Model file for the job. Use its own axes, mm. Face numbers are marked on the shaded views. A direction names the side the tool comes from. Round coordinates to 2 decimals unless told otherwise and drop trailing zeros. Loops run counter-clockwise (first coordinate to the right, second up) from the corner with the lowest first, then second, coordinate; pieces in that order, holes last. Notation, with made-up numbers: M 24,24.25 L 59,24.25 A20 cw 59,57.25 Z; hole C 4,-4.5 d5. An arc over 180 degrees is marked long. Answer in a Markdown table with one row per item.
from build123d import *

# Parameters (mm, degrees)
SKETCH_1_R          = 8
EXTRUDE_1_DEPTH     = 6
SKETCH_2_R          = 1.25
CUT_EXTRUDE_1_DEPTH = 3


with BuildPart() as part:
    # 草图1 → 凸台-拉伸1 (new body)
    with BuildSketch(Plane.XY):
        with BuildLine():
            Line((-3, -30), (-18, -30))
            Line((-18, -30), (-18, -27))
            Line((-18, -27), (-11.5, -27))
            Line((-11.5, -27), (-11.5, 0))
            ThreePointArc((-11.5, 0), (0, 11.5), (11.5, 0))
            Line((11.5, 0), (11.5, -27))
            Line((11.5, -27), (17.5, -27))
            Line((17.5, -27), (17.5, -30))
            Line((17.5, -30), (3, -30))
            Line((3, -30), (3, -33))
            Line((3, -33), (0, -33))
            Line((0, -33), (-3, -33))
            Line((-3, -33), (-3, -30))
        make_face()
        Circle(SKETCH_1_R, mode=Mode.SUBTRACT)
    extrude(amount=EXTRUDE_1_DEPTH)

    # 草图2 → 切除-拉伸1 (cut)
    with BuildSketch(Plane(origin=(0, -27, 0), x_dir=(1, 0, 0), z_dir=(0, 1, 0))):
        with Locations(Location((-14.5, -3, 0), (0, 0, 270))):
            Circle(SKETCH_2_R)
        with Locations(Location((14.5, -3, 0), (0, 0, 270))):
            Circle(SKETCH_2_R)
    extrude(amount=-CUT_EXTRUDE_1_DEPTH, mode=Mode.SUBTRACT)


solid = part.part
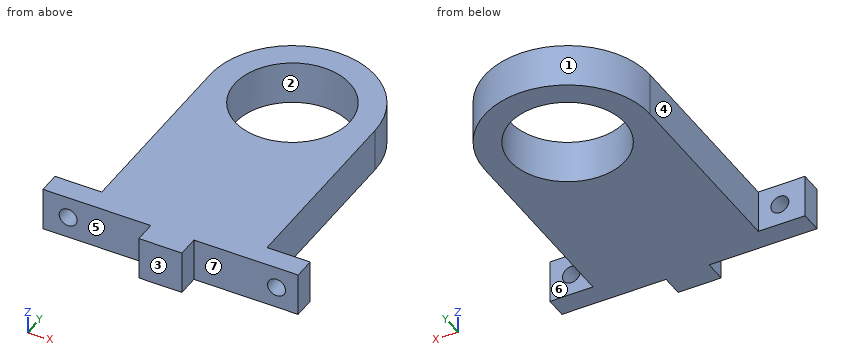
1. Wall check: probe 1 along X at (y, z) = (-29.3, 3); probe 2 along Y at (x, z) = (0, 3.25); probe 3 along X at (y, z) = (-25, 3.05). Give the ranges that are in metal, low to high.
Verdict:
| item | result |
|---|---|
| probe 1 | x = -18 to -15.75, -13.25 to 13.25, 15.75 to 17.5 |
| probe 2 | y = -33 to -8, 8 to 11.5 |
| probe 3 | x = -11.5 to 11.5 |
2. Mould opens along X. For the marked faces 1, 2 and 3 say: +X half, -X half, draft (parallel to the pull), parting line (faces both ways), or undercut.
Verdict:
| item | result |
|---|---|
| face 1 | parting line |
| face 2 | undercut |
| face 3 | draft |
3. Saw through at B-B (x = 0). Write the cut outline in (y, z).
Verdict:
| item | result |
|---|---|
| outline | M -33,0 L -8,0 L -8,6 L -33,6 Z; M 8,0 L 11.5,0 L 11.5,6 L 8,6 Z |
4. Saw through at A-A (z = 3). Write the cut outline in (x, y), and give its area (3 significant figures).
Verdict:
| item | result |
|---|---|
| outline | M -18,-30 L -15.75,-30 L -15.75,-27 L -18,-27 Z; M -13.25,-30 L -3,-30 L -3,-33 L 3,-33 L 3,-30 L 13.25,-30 L 13.25,-27 L 11.5,-27 L 11.5,0 A11.5 ccw -11.5,0 L -11.5,-27 L -13.25,-27 Z; M 15.75,-30 L 17.5,-30 L 17.5,-27 L 15.75,-27 Z; hole C 0,0 d16 |
| area | 737 mm² |
5. Saw through at D-D (y = -18.5). Write the cut outline in (x, z), and give its area (3 significant figures).
Verdict:
| item | result |
|---|---|
| outline | M -11.5,0 L 11.5,0 L 11.5,6 L -11.5,6 Z |
| area | 138 mm² |
6. Tool access for the marked faces 4, 5, 6 and 7: list every direction of +Z, -Z, +X, -X, +Y, -Y with a clear straight run to the whole face (end or side of a thin tool).
Verdict:
| item | result |
|---|---|
| face 4 | +Z, -Z, -X, +Y |
| face 5 | +Z, -Z, -X, -Y |
| face 6 | +Z, -Z, +X, +Y |
| face 7 | +Z, -Z, +X, -Y |
7. Saw through at C-C (y = -7). Write the cut outline in (x, z).
Verdict:
| item | result |
|---|---|
| outline | M -11.5,0 L -3.87,0 L -3.87,6 L -11.5,6 Z; M 3.87,0 L 11.5,0 L 11.5,6 L 3.87,6 Z |
8. Pin check, flat tips, straight feed: pin 1 (1.5 mm diameter, centred on y = -31.5, z = 3.5, fed in from +X); pin 2 (0.9 mm diameter, centred on y = -31, z = 4, fed in from -X); pin 3 (2 mm diameter, centred on y = -11.5, z = 5, fed in from -X). Stop position of each tip, or through.
Verdict:
| item | result |
|---|---|
| pin 1 | stops at x = 3 |
| pin 2 | stops at x = -3 |
| pin 3 | stops at x = -11.5 |
